Autodesk Fusion 360 part; units mm, degrees
sketch "スケッチ4" plane through (0, 0, 0) normal (0, 0, 1) x (1, 0, 0) in component "Component"
  arc A0 (-6.9712, -3.9246) -> (-6.9712, 3.9246) centre (0, 0) ccw
  line L0 (-6.9712, 0.9595) -> (-0.9758, 0.9595)
  line L1 (-0.9758, 0.9595) -> (-0.9758, -1.0395)
  line L2 (-0.9758, -1.0395) -> (-6.9712, -1.0395)
  line L3 (-6.9712, 3.9246) -> (-6.9712, 0.9595)
  line L4 (-6.9712, -1.0395) -> (-6.9712, -3.9246)
  dimension "d29" = 16
extrude "押し出し1" add sketch "スケッチ4" along normal blind 14 makes body 1 in component "Component"
cylinder "円柱プリミティブ1" add diameter 11 height 6 placed x (0, 0, -1) y (0, 1, 0) z (1, 0, 0) at (0, 23.0583, 6.8926) separate body makes body 2
move_body "移動1" bodies 2 to x (1, 0, 0) y (0, 1, 0) z (0, 0, 1) at (0, -23.0583, -6.8926)
move_body "移動2" bodies 2 to x (1, 0, 0) y (0, 1, 0) z (0, 0, 1) at (3, 0, 7)
combine "結合2" operation add target body 1 tool bodies 2 in component "Component"
hole "穴4" at (0, 0, 14) direction (0, 0, -1) diameter 13.5 depth 15 tip angle 180 bodies 1 in component "Component"
hole "穴6" at (9, 0, 7) direction (-1, 0, 0) diameter 10 depth 1.5 tip angle 180 bodies 1 in component "Component"
fillet "フィレット4" radius 0.625 4 edges at (8, 0, 14) (6.7499, 0.0404, 14) (8, 0, 0) (6.7499, 0.0404, 0) on bodies 1 in component "Component"
component "Component" placed x (1, 0, 0) y (0, 1, 0) z (0, 0, 1) at (0, 0, 0)
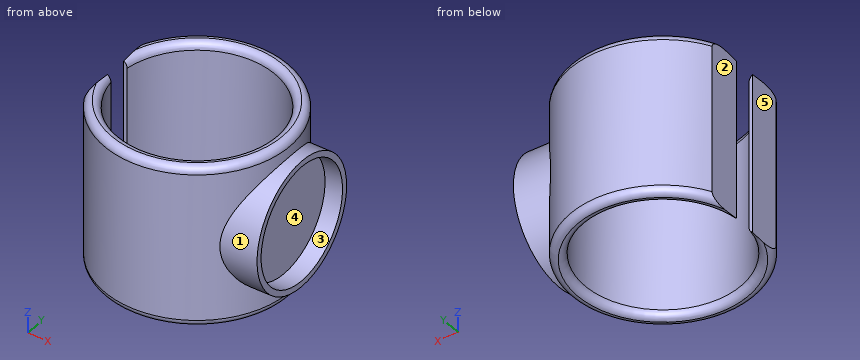
Design review of the part built by this model. Coordinates are the model's own, in mm. Face numbers are marked on the shaded views. A direction names the side the tool comes from. Round coordinates to 2 decimals unless told otherwise and drop trailing zeros. Write each loop counter-clockwise with the first axis right and the second up, starting at its lowest first coordinate (ties: lowest second). Pieces come first, ordered by that corner, then holes. Notation, with made-up numbers: (4.25, 1.25) -> (23.25, 1.25) arc R16 cw to (23.25, 19.25) -> close; hole circle Ø8 at (57, 37). An arc over 180 degrees is marked (long way). Write item = value, one per line. Start each with the question number.
1) Mouldability with a two-part tool opening along Y and no side actions: class the marked faces 1, 2 and 3 as +Y half, -Y half, draft (parallel to the pull), parting line (faces both ways), or undercut.
2) Wall thickness on probe 1 along Y at (x, z) = (8.4, 7); probe 2 along X at (y, z) = (0, 5); probe 3 along Y at (x, z) = (1, 11.75): over which ranges is each line inside the solid? List them lowest first. Write a range as from..to.
3) Tool access review of the marked faces 4 and 5: name each direction out of +Z, -Z, +X, -X, +Y, -Y from which nothing blocks a thin tool from reaching the whole face with its end or side.
4) Take a section at A-A, the plane z = 7. State the section outline as (x, y) points, plus the area to 3 significant figures.
5) Clearance check with flat-ended pins moving along their axes: pin 1 (2 mm diameter, centred on x = -1.5, z = 10.5, fed in from -Y); pin 2 (1 mm diameter, centred on x = 2.5, z = 5, fed in from -Y); pin 3 (3 mm diameter, centred on x = -4.5, z = 11.5, fed in from +Y). State where each tip first meets the part, or that it passes through.
Results list:
q1.face_1 = parting line
q1.face_2 = draft
q1.face_3 = undercut
q2.probe_1 = -5.5..-5, 5..5.5
q2.probe_2 = 6.75..7.5
q2.probe_3 = -7.94..-6.68, 6.68..7.94
q3.face_4 = +X
q3.face_5 = +Z, -Z, -X, +Y, -Y
q4.outline = (-6.97, -3.92) arc R8 ccw to (5.81, -5.5) -> (9, -5.5) -> (9, -5) -> (7.5, -5) -> (7.5, 5) -> (9, 5) -> (9, 5.5) -> (5.81, 5.5) arc R8 ccw to (-6.97, 3.92) -> (-6.97, 0.96) -> (-6.68, 0.96) arc R6.75 cw (long way) to (-6.67, -1.04) -> (-6.97, -1.04) -> close
q4.area = 55.5 mm²
q5.pin_1 = -7.98
q5.pin_2 = -7.75
q5.pin_3 = 7.42
